```python
from build123d import *

# Parameters (mm, degrees)
F1_DEPTH = 19.05
F2_R     = 0.508
F4_DEPTH = 25.4
F6_DEPTH = 25.4


with BuildPart() as f1:
    # F0 (on Front) → F1 (new body)
    with BuildSketch(Plane.XZ):
        Polygon((-25.6741352886, 34.6823864549), (-27.2616352886, 34.6823864549), (-27.2616352886, 14.0448864549), (-6.6241352886, 14.0448864549), (-6.6241352886, 15.6323864549), (-25.6741352886, 15.6323864549), align=None)
    extrude(amount=F1_DEPTH)

    # F2
    f2_edges = [f1.edges().sort_by_distance(p)[0] for p in [
        (-27.261635, -9.525, 14.044886),
        (-27.261635, -9.525, 34.682386),
        (-25.674135, -9.525, 34.682386),
        (-6.624135, -9.525, 15.632386),
        (-25.674135, -9.525, 15.632386),
    ]]
    fillet(f2_edges, radius=F2_R)

    # F3 (on face) → F4 (cut)
    with BuildSketch(Plane(origin=(-27.2616352886, 0, 0), x_dir=(0, -1, 0), z_dir=(-1, 0, 0))):
        with BuildLine():
            Line((4.7625, 24.3636364549), (14.2875, 24.3636364549))
            ThreePointArc((14.2875, 24.3636364549), (9.525, 29.1261364549), (4.7625, 24.3636364549))
        make_face()
        with BuildLine():
            ThreePointArc((4.7625, 24.3636364549), (9.525, 19.6011364549), (14.2875, 24.3636364549))
            Line((14.2875, 24.3636364549), (4.7625, 24.3636364549))
        make_face()
    extrude(amount=-F4_DEPTH, mode=Mode.SUBTRACT)

    # F5 (on face) → F6 (cut)
    with BuildSketch(Plane.XY.offset(15.6323864549)):
        with BuildLine():
            Line((-20.9116352886, -9.525), (-11.3866352886, -9.525))
            ThreePointArc((-11.3866352886, -9.525), (-16.1491352886, -4.7625), (-20.9116352886, -9.525))
        make_face()
        with BuildLine():
            ThreePointArc((-20.9116352886, -9.525), (-16.1491352886, -14.2875), (-11.3866352886, -9.525))
            Line((-11.3866352886, -9.525), (-20.9116352886, -9.525))
        make_face()
    extrude(amount=-F6_DEPTH, mode=Mode.SUBTRACT)


solid = f1.part
```
The model under review builds one solid part; all positions refer to its coordinate system, in mm. A direction names the side the tool comes from. Give positions to 0.01 mm unless a question says otherwise; leave off trailing zeros. Loops run counter-clockwise (first coordinate to the right, second up) from the corner with the lowest first, then second, coordinate; pieces in that order, holes last. Notation, with made-up numbers: (-25, 17.5) -> (25, 17.5) arc R20 cw to (25, 27.5) -> close; hole circle Ø2 at (29, 62.5). An arc over 180 degrees is marked (long way). Use CSV: the item, a comma, the result in double quotes.
1. Consider section A-A, the plane x = -12. Write out the cut boundary in (y, z), then the cut area to 3 significant figures.
Result:
outline,"(-19.05, 14.04) -> (-11.86, 14.04) -> (-11.86, 15.63) -> (-19.05, 15.63) -> close; (-7.19, 14.04) -> (0, 14.04) -> (0, 15.63) -> (-7.19, 15.63) -> close"
area,"22.8 mm²"
2. To check wall thickness, follow probe 1 along Z at (x, y) = (-24, -10.5); probe 2 along X at (y, z) = (-2.75, 18.25); probe 3 along Y at (x, z) = (-17.5, 15.5). State the ranges of each line that lie inside material, in increasing order. Write a range as from..to.
Result:
probe 1,"z = 14.04..15.63"
probe 2,"x = -27.26..-25.67"
probe 3,"y = -19.05..-14.09, -4.96..0"
3. Consider section B-B, the plane z = 22.25. Write out the cut boundary in (x, y).
Result:
outline,"(-27.26, -19.05) -> (-25.67, -19.05) -> (-25.67, -13.79) -> (-27.26, -13.79) -> close; (-27.26, -5.26) -> (-25.67, -5.26) -> (-25.67, 0) -> (-27.26, 0) -> close"
4. For P1, Ø8, axis at y = -17, z = 29.5, coming from the +X side; P2, Ø6, axis at x = -19, y = -11.5, coming from the -Z side; P3, Ø5, axis at x = -12.5, y = -6.5, coming from the +Z side, all flat-tipped, find the tip position at first contact; note any pin that passes through.
Result:
P1,"stops at x = -25.67"
P2,"stops at z = 14.04"
P3,"stops at z = 15.63"
5. The part is to be moulded in two halves that separate along Y. For faces 1 (the face through (-26, 0, 20)), 2 (the face through (-21.3, -9.4, 14.045)), 3 (the face through (-26.479, -13.304, 27.262)), say which applies: +Y half, -Y half, draft (parallel to the pull), parting line (faces both ways), or undercut.
Result:
face 1,"+Y half"
face 2,"draft"
face 3,"undercut"
6. Machinability: for faces 4 (the face through (-25.674, -12, 29)), 5 (the face through (-18.35, -5.3, 14.85)), which of the approach directions +Z, -Z, +X, -X, +Y, -Y give a long, thin tool a straight path to every point of the face, cutting with its end or side? Answer none if there is none.
Result:
face 4,"+Z, +X, +Y, -Y"
face 5,"+Z, -Z"
7. Consider section C-C, the plane y = -11.25. Write out the cut boundary in (x, z), then the cut area to 3 significant figures.
Result:
outline,"(-27.26, 14.55) arc R0.51 ccw to (-26.75, 14.04) -> (-20.59, 14.04) -> (-20.59, 15.63) -> (-25.17, 15.63) arc R0.51 cw to (-25.67, 16.14) -> (-25.67, 19.92) -> (-27.26, 19.92) -> close; (-27.26, 28.8) -> (-25.67, 28.8) -> (-25.67, 34.17) arc R0.51 ccw to (-26.18, 34.68) -> (-26.75, 34.68) arc R0.51 ccw to (-27.26, 34.17) -> close; (-11.71, 14.04) -> (-6.62, 14.04) -> (-6.62, 15.12) arc R0.51 ccw to (-7.13, 15.63) -> (-11.71, 15.63) -> close"
area,"34.6 mm²"
8. Consider section D-D, the plane y = -17. Write out the cut boundary in (x, z), then the cut area to 3 significant figures.
Result:
outline,"(-27.26, 14.55) arc R0.51 ccw to (-26.75, 14.04) -> (-6.62, 14.04) -> (-6.62, 15.12) arc R0.51 ccw to (-7.13, 15.63) -> (-25.17, 15.63) arc R0.51 cw to (-25.67, 16.14) -> (-25.67, 34.17) arc R0.51 ccw to (-26.18, 34.68) -> (-26.75, 34.68) arc R0.51 ccw to (-27.26, 34.17) -> close"
area,"62.8 mm²"
